Answer from the drawing. Dimensions are ordinates in mm from the lowest x, y and z of the part. A direction names the side the tool comes from. Round coordinates to 2 decimals unless told otherwise and drop trailing zeros. Write each loop counter-clockwise with the first axis right and the second up, starting at its lowest first coordinate (ties: lowest second). Pieces come first, ordered by that corner, then holes.
1. Find section C-C (z = 3.5). Write down the section's boundary in (x, y).
2. Determine the mould class of the marked faces 3, 4 and 5 for opening direction X: pulls with the +X half, pulls with the -X half, needs draft (parallel to the pull), parting line crosses it, or undercut.
3. Straight lines are drawn through the part: probe 1 along Z at (x, y) = (10.5, 6.25); probe 2 along Z at (x, y) = (13, 1); probe 3 along X at (y, z) = (12.5, 6) (1 decimal). For each, find the intervals that lie inside material, in ascending order.
4. Find section B-B (x = 6). Write down the section's boundary in (y, z).
5. Find section D-D (y = 15.5). Write down the section's boundary in (x, z) (1 decimal), and give its area (3 significant figures).
6. A tool of negligible diameter and unlimited length cuts with its end or side. For the marked faces 1 and 2, from which of +Z, -Z, +X, -X, +Y, -Y can it reach the whole face along a straight path? Write none if from no direction.
7. Flat-ended cylindrical pins translate along their axes: pin 1 Ø1.5 at (x, z) = (13, 4) entering from +Y; pin 2 Ø1.5 at (y, z) = (16, 2.5) entering from -X. Find the tip coordinate at first contact, or state that the pin passes through.
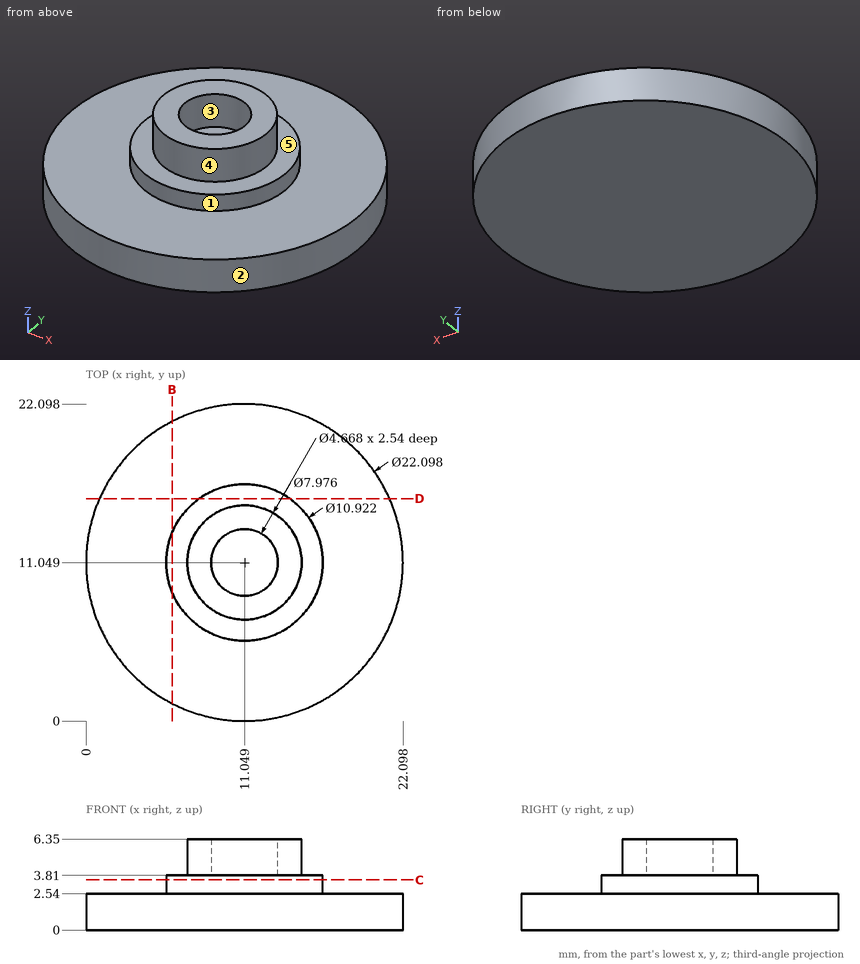
Worked answers:
1. outline: circle Ø10.92 at (11.05, 11.05)
2. face 3: undercut
2. face 4: parting line crosses it
2. face 5: needs draft
3. probe 1: z = 0 to 3.81
3. probe 2: z = 0 to 2.54
3. probe 3: x = 7.3 to 9.2, 12.9 to 14.8
4. outline: (1.22, 0) - (20.88, 0) - (20.88, 2.54) - (13.13, 2.54) - (13.13, 3.81) - (8.97, 3.81) - (8.97, 2.54) - (1.22, 2.54) - close
5. outline: (0.9, 0) - (21.2, 0) - (21.2, 2.5) - (14.2, 2.5) - (14.2, 3.8) - (7.9, 3.8) - (7.9, 2.5) - (0.9, 2.5) - close
5. area: 59.4 mm2
6. face 1: +Z
6. face 2: +Z, -Z
7. pin 1: stops at y = 16.37
7. pin 2: stops at x = 0.83
